Check sheet for the drawn part. Datum: minimum x, y, z corner. Units: mm. Coordinates: 2 decimals unless noted, no trailing zeros. Order: outer loops, then holes, each group sorted by start corner. A loop starts at its lowest first (then second) coordinate and runs counter-clockwise, first axis right, second up. Notation, with made-up numbers: (-10.75, 38.5) - (-6.75, 38.5) arc R25 cw to (-6.75, 68.5) - close; hole circle Ø3 at (38.5, 71.25). An arc over 180 degrees is marked (long way). Return JSON: item names as keys, results as strings. Group by question number.
Item 1: Scan lines: probe 1 along X at (y, z) = (0.5, 50); probe 2 along X at (y, z) = (0.3, 52); probe 3 along Z at (x, y) = (42, 0.5) (1 decimal). Record each from-to range of solid material in increasing order.
Item 2: Section check B-B on y = 0.75. Enter the section's corners in (x, z) (1 decimal), then the cut area to 3 significant figures.
Item 3: Gauge pin test, flat ends, axial feed: pin 1 (4 mm diameter, centred on x = 63.02, z = 50, fed in from -Y); pin 2 (8 mm diameter, centred on x = 42.6, z = 50, fed in from -Y). Record the tip position at first contact, or that the pin passes through.
Item 4: Section check D-D on x = 23. Enter the section's corners in (y, z).
Item 5: Section check C-C on x = 63.02. Enter the section's corners in (y, z).
Item 6: Section check A-A on z = 50. Enter the section's corners in (x, y).
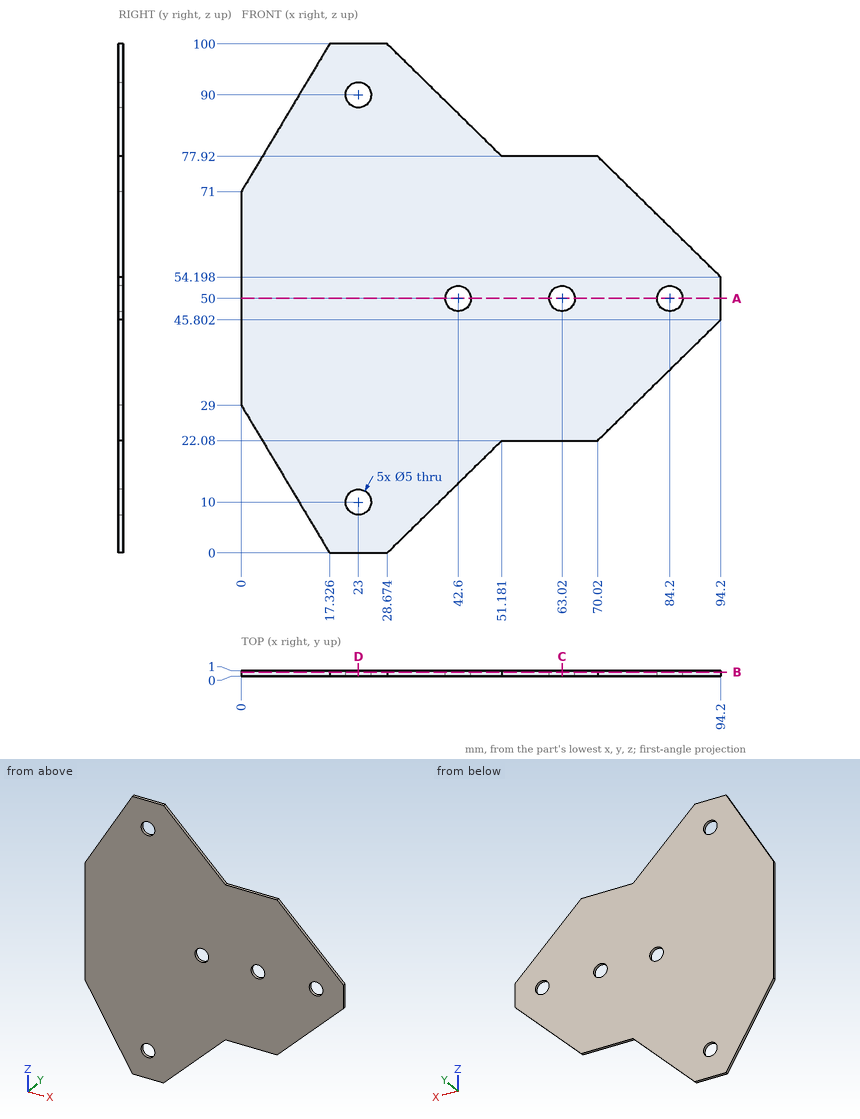
Computed:
{
 "1": {"probe 1": "x = 0 to 40.1, 45.1 to 60.52, 65.52 to 81.7, 86.7 to 94.2", "probe 2": "x = 0 to 41.1, 44.1 to 61.52, 64.52 to 82.7, 85.7 to 94.2", "probe 3": "z = 13.1 to 47.6, 52.4 to 86.9"},
 "2": {"outline": "(0, 29) - (17.3, 0) - (28.7, 0) - (51.2, 22.1) - (70, 22.1) - (94.2, 45.8) - (94.2, 54.2) - (70, 77.9) - (51.2, 77.9) - (28.7, 100) - (17.3, 100) - (0, 71) - close; hole circle Ø5 at (23, 10); hole circle Ø5 at (23, 90); hole circle Ø5 at (42.6, 50); hole circle Ø5 at (63, 50); hole circle Ø5 at (84.2, 50)", "area": "5,850 mm²"},
 "3": {"pin 1": "passes through", "pin 2": "stops at y = 0"},
 "4": {"outline": "(0, 0) - (1, 0) - (1, 7.5) - (0, 7.5) - close; (0, 12.5) - (1, 12.5) - (1, 87.5) - (0, 87.5) - close; (0, 92.5) - (1, 92.5) - (1, 100) - (0, 100) - close"},
 "5": {"outline": "(0, 22.08) - (1, 22.08) - (1, 47.5) - (0, 47.5) - close; (0, 52.5) - (1, 52.5) - (1, 77.92) - (0, 77.92) - close"},
 "6": {"outline": "(0, 0) - (40.1, 0) - (40.1, 1) - (0, 1) - close; (45.1, 0) - (60.52, 0) - (60.52, 1) - (45.1, 1) - close; (65.52, 0) - (81.7, 0) - (81.7, 1) - (65.52, 1) - close; (86.7, 0) - (94.2, 0) - (94.2, 1) - (86.7, 1) - close"}
}
